```python
from build123d import *

# Parameters (mm, degrees)
CROQUIS1_R              = 2.6
SALIENTE_EXTRUIR1_DEPTH = 10
CROQUIS5_R              = 4
CORTAR_EXTRUIR2_DEPTH   = 5
FILLET1_R               = 3
SKETCH1_R               = 4
CUT_EXTRUDE1_DEPTH      = 5


with BuildPart() as part:
    # Croquis1 → Saliente-Extruir1 (new body)
    with BuildSketch(Plane(origin=(0, 0, 0), x_dir=(0, 0, -1), z_dir=(1, 0, 0))):
        Polygon((-25, -120), (25, -120), (25, 25), (0, 25), (-25, 25), (-25, 0), align=None)
        with Locations((-17.68, 17.68)):
            Circle(CROQUIS1_R, mode=Mode.SUBTRACT)
        with Locations(Location((17.68, 17.68, 0), (0, 0, 180))):
            Circle(CROQUIS1_R, mode=Mode.SUBTRACT)
        with Locations((17.68, -17.68)):
            Circle(CROQUIS1_R, mode=Mode.SUBTRACT)
        with Locations(Location((-17.68, -17.68, 0), (0, 0, 180))):
            Circle(CROQUIS1_R, mode=Mode.SUBTRACT)
        with Locations((-17.68, -115)):
            Circle(CROQUIS1_R, mode=Mode.SUBTRACT)
        with Locations(Location((17.68, -115, 0), (0, 0, 180))):
            Circle(CROQUIS1_R, mode=Mode.SUBTRACT)
    extrude(amount=SALIENTE_EXTRUIR1_DEPTH)

    # Croquis5 → Cortar-Extruir2 (cut)
    with BuildSketch(Plane(origin=(10, 0, 0), x_dir=(0, 0, -1), z_dir=(1, 0, 0))):
        with Locations((17.68, 17.68)):
            Circle(CROQUIS5_R)
        with Locations((-17.68, 17.68)):
            Circle(CROQUIS5_R)
        with Locations((-17.68, -17.68)):
            Circle(CROQUIS5_R)
        with Locations((17.68, -17.68)):
            Circle(CROQUIS5_R)
    extrude(amount=-CORTAR_EXTRUIR2_DEPTH, mode=Mode.SUBTRACT)

    # Fillet1
    fillet1_edges = [part.edges().sort_by_distance(p)[0] for p in [
        (5, 25, -25),
        (5, 25, 25),
    ]]
    fillet(fillet1_edges, radius=FILLET1_R)

    # Sketch1 → Cut-Extrude1 (cut)
    with BuildSketch(Plane.ZY):
        with Locations((17.68, -115)):
            Circle(SKETCH1_R)
        with Locations(Location((-17.68, -115, 0), (0, 0, 180))):
            Circle(SKETCH1_R)
    extrude(amount=-CUT_EXTRUDE1_DEPTH, mode=Mode.SUBTRACT)


solid = part.part
```
Could you check a few things on this model? Use its own coordinates, in mm. A direction names the side the tool comes from. Round coordinates to 2 decimals unless told otherwise and drop trailing zeros. Write each loop counter-clockwise with the first axis right and the second up, starting at its lowest first coordinate (ties: lowest second). Pieces come first, ordered by that corner, then holes. Notation, with made-up numbers: M 63,38.25 L 73,38.25 A22 ccw 73,62.25 Z; hole C -32.75,-33 d4. An arc over 180 degrees is marked long. Write each question's results on one line, items separated by ' | '. Start each with the question number.
1. Imagine slicing it at A-A on x = 2.75. List the corners of the cut face in (y, z) for me.
2. On a 3-axis mill with a long thin cutter (end or side, diameter ignored), from which of +Z, -Z, +X, -X, +Y, -Y can I reach the whole of each face in a straight line? I mean faces 1 (the face through (7.54, 20.38, -14.73)), 2 (the face through (5.07, 24.1, -24.14)), 3 (the face through (2.465, -111.034, 17.159)). Say none if no direction works.
3. Imagine slicing it at C-C on y = -115. List the corners of the cut face in (x, z) for me.
4. I'm going to push flat-ended pins straight in: pin 1 Ø4 at (y, z) = (-17.5, -18.5) entering from +X; pin 2 Ø2.5 at (y, z) = (-116.5, 16) entering from -X. Where does each tip first touch, or does it pass through?
5. I need wall thicknesses on L1, parallel to Z at x = 1.1, y = 17.68; L2, parallel to Y at x = 3.3, z = -17.68; L3, parallel to Y at x = 7.7, z = 17.68. Which ranges of each line are inside material? Lowest first, please. Write a range as from..to.
6. Imagine slicing it at B-B on z = -17.68. List the corners of the cut face in (x, y) for me, and give its area (3 significant figures).
Result sheet:
1) outline: M -120,-25 L 22,-25 A3 ccw 25,-22 L 25,22 A3 ccw 22,25 L -120,25 Z; hole C -115,-17.68 d8; hole C -115,17.68 d8; hole C -17.68,-17.68 d5.2; hole C -17.68,17.68 d5.2; hole C 17.68,-17.68 d5.2; hole C 17.68,17.68 d5.2
2) face 1: +X | face 2: -Z, +X, -X, +Y | face 3: -X
3) outline: M 0,-25 L 10,-25 L 10,-20.28 L 5,-20.28 L 5,-21.68 L 0,-21.68 Z; M 0,-13.68 L 5,-13.68 L 5,-15.08 L 10,-15.08 L 10,15.08 L 5,15.08 L 5,13.68 L 0,13.68 Z; M 0,21.68 L 5,21.68 L 5,20.28 L 10,20.28 L 10,25 L 0,25 Z
4) pin 1: stops at x = 5 | pin 2: stops at x = 5
5) L1: z = -25..-20.28, -15.08..15.08, 20.28..25 | L2: y = -120..-119, -111..-20.28, -15.08..15.08, 20.28..25 | L3: y = -120..-117.6, -112.4..-21.68, -13.68..13.68, 21.68..25
6) outline: M 0,-120 L 10,-120 L 10,-117.6 L 5,-117.6 L 5,-119 L 0,-119 Z; M 0,-111 L 5,-111 L 5,-112.4 L 10,-112.4 L 10,-21.68 L 5,-21.68 L 5,-20.28 L 0,-20.28 Z; M 0,-15.08 L 5,-15.08 L 5,-13.68 L 10,-13.68 L 10,13.68 L 5,13.68 L 5,15.08 L 0,15.08 Z; M 0,20.28 L 5,20.28 L 5,21.68 L 10,21.68 L 10,25 L 0,25 Z | area: 1,250 mm^2
